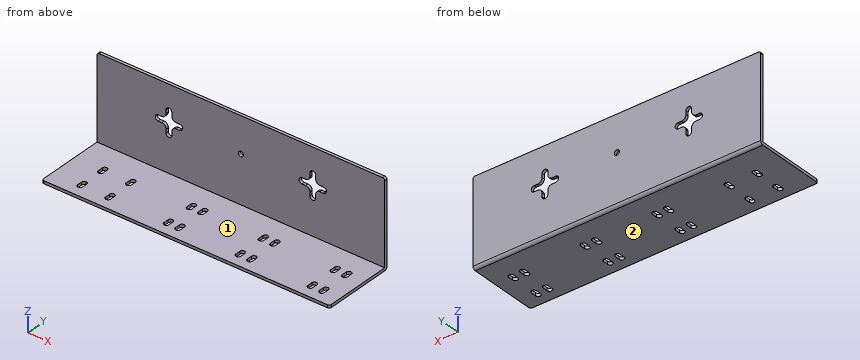
from build123d import *

# Parameters (mm, degrees)
F1_DEPTH = 100
F3_DEPTH = 60.001
F4_R     = 1.5
F5_R     = 2
F6_R     = 1.75
F6_W     = 2
F6_H     = 2
F7_DEPTH = 2
F8_R     = 3


with BuildPart() as f1:
    # F0 (on Right) → F1 (new body, symmetric)
    with BuildSketch(Plane.YZ):
        Polygon((0, 2), (0, 0), (50, 0), (50, 60), (48, 60), (48, 2), align=None)
    extrude(amount=F1_DEPTH, both=True)

    # F2 (on face) → F3 (cut, through all)
    with BuildSketch(Plane(origin=(0, 0, 0), x_dir=(1, 0, 0), z_dir=(0, 0, -1))):
        with BuildLine():
            Line((-18.25, -11.75), (-18.25, -10))
            Line((-18.25, -10), (-18.25, -8.25))
            ThreePointArc((-18.25, -8.25), (-20, -6.5), (-21.75, -8.25))
            Line((-21.75, -8.25), (-21.75, -11.75))
            ThreePointArc((-21.75, -11.75), (-20, -13.5), (-18.25, -11.75))
        make_face()
        with BuildLine():
            Line((-13.75, -8.25), (-13.75, -10))
            Line((-13.75, -10), (-13.75, -11.75))
            ThreePointArc((-13.75, -11.75), (-12, -13.5), (-10.25, -11.75))
            Line((-10.25, -11.75), (-10.25, -8.25))
            ThreePointArc((-10.25, -8.25), (-12, -6.5), (-13.75, -8.25))
        make_face()
        with BuildLine():
            ThreePointArc((-21.75, -31.75), (-20, -33.5), (-18.25, -31.75))
            Line((-18.25, -31.75), (-18.25, -28.25))
            ThreePointArc((-18.25, -28.25), (-20, -26.5), (-21.75, -28.25))
            Line((-21.75, -28.25), (-21.75, -31.75))
        make_face()
        with BuildLine():
            Line((-10.25, -31.75), (-10.25, -28.25))
            ThreePointArc((-10.25, -28.25), (-12, -26.5), (-13.75, -28.25))
            Line((-13.75, -28.25), (-13.75, -31.75))
            ThreePointArc((-13.75, -31.75), (-12, -33.5), (-10.25, -31.75))
        make_face()
        with BuildLine():
            Line((31.75, -10), (31.75, -8.25))
            ThreePointArc((31.75, -8.25), (30, -6.5), (28.25, -8.25))
            Line((28.25, -8.25), (28.25, -11.75))
            ThreePointArc((28.25, -11.75), (30, -13.5), (31.75, -11.75))
            Line((31.75, -11.75), (31.75, -10))
        make_face()
        with BuildLine():
            Line((39.75, -11.75), (39.75, -8.25))
            ThreePointArc((39.75, -8.25), (38, -6.5), (36.25, -8.25))
            Line((36.25, -8.25), (36.25, -10))
            Line((36.25, -10), (36.25, -11.75))
            ThreePointArc((36.25, -11.75), (38, -13.5), (39.75, -11.75))
        make_face()
        with BuildLine():
            Line((39.75, -31.75), (39.75, -28.25))
            ThreePointArc((39.75, -28.25), (38, -26.5), (36.25, -28.25))
            Line((36.25, -28.25), (36.25, -31.75))
            ThreePointArc((36.25, -31.75), (38, -33.5), (39.75, -31.75))
        make_face()
        with BuildLine():
            ThreePointArc((28.25, -31.75), (30, -33.5), (31.75, -31.75))
            Line((31.75, -31.75), (31.75, -28.25))
            ThreePointArc((31.75, -28.25), (30, -26.5), (28.25, -28.25))
            Line((28.25, -28.25), (28.25, -31.75))
        make_face()
        with BuildLine():
            Line((81.75, -10), (81.75, -8.25))
            ThreePointArc((81.75, -8.25), (80, -6.5), (78.25, -8.25))
            Line((78.25, -8.25), (78.25, -11.75))
            ThreePointArc((78.25, -11.75), (80, -13.5), (81.75, -11.75))
            Line((81.75, -11.75), (81.75, -10))
        make_face()
        with BuildLine():
            Line((89.75, -11.75), (89.75, -8.25))
            ThreePointArc((89.75, -8.25), (88, -6.5), (86.25, -8.25))
            Line((86.25, -8.25), (86.25, -10))
            Line((86.25, -10), (86.25, -11.75))
            ThreePointArc((86.25, -11.75), (88, -13.5), (89.75, -11.75))
        make_face()
        with BuildLine():
            ThreePointArc((78.25, -31.75), (80, -33.5), (81.75, -31.75))
            Line((81.75, -31.75), (81.75, -28.25))
            ThreePointArc((81.75, -28.25), (80, -26.5), (78.25, -28.25))
            Line((78.25, -28.25), (78.25, -31.75))
        make_face()
        with BuildLine():
            Line((89.75, -31.75), (89.75, -28.25))
            ThreePointArc((89.75, -28.25), (88, -26.5), (86.25, -28.25))
            Line((86.25, -28.25), (86.25, -31.75))
            ThreePointArc((86.25, -31.75), (88, -33.5), (89.75, -31.75))
        make_face()
        with BuildLine():
            ThreePointArc((-81.75, -11.75), (-81.2374368671, -12.9874368671), (-80, -13.5))
            ThreePointArc((-80, -13.5), (-78.7625631329, -12.9874368671), (-78.25, -11.75))
            Line((-78.25, -11.75), (-78.25, -8.25))
            ThreePointArc((-78.25, -8.25), (-80, -6.5), (-81.75, -8.25))
            Line((-81.75, -8.25), (-81.75, -11.75))
        make_face()
        with BuildLine():
            Line((-78.25, -29.75), (-78.25, -28))
            Line((-78.25, -28), (-78.25, -26.25))
            ThreePointArc((-78.25, -26.25), (-78.7625631329, -25.0125631329), (-80, -24.5))
            ThreePointArc((-80, -24.5), (-81.2374368671, -25.0125631329), (-81.75, -26.25))
            Line((-81.75, -26.25), (-81.75, -29.75))
            ThreePointArc((-81.75, -29.75), (-80, -31.5), (-78.25, -29.75))
        make_face()
        with BuildLine():
            Line((-62.35, -26.25), (-62.35, -28))
            Line((-62.35, -28), (-62.35, -29.75))
            ThreePointArc((-62.35, -29.75), (-60.6, -31.5), (-58.85, -29.75))
            Line((-58.85, -29.75), (-58.85, -26.25))
            ThreePointArc((-58.85, -26.25), (-60.6, -24.5), (-62.35, -26.25))
        make_face()
        with BuildLine():
            Line((-62.35, -10), (-62.35, -11.75))
            ThreePointArc((-62.35, -11.75), (-60.6, -13.5), (-58.85, -11.75))
            Line((-58.85, -11.75), (-58.85, -8.25))
            ThreePointArc((-58.85, -8.25), (-60.6, -6.5), (-62.35, -8.25))
            Line((-62.35, -8.25), (-62.35, -10))
        make_face()
    extrude(amount=-F3_DEPTH, mode=Mode.SUBTRACT)

    # F4
    f4_edges = [f1.edges().sort_by_distance(p)[0] for p in [
        (100, 0, 1),
        (100, 49, 60),
        (-100, 0, 1),
        (-100, 49, 60),
    ]]
    fillet(f4_edges, radius=F4_R)

    # F5
    f5_edges = [f1.edges().sort_by_distance(p)[0] for p in [
        (0, 50, 0),
    ]]
    fillet(f5_edges, radius=F5_R)

    # F6 (on face) → F7 (cut)
    with BuildSketch(Plane(origin=(0, 50, 0), x_dir=(-1, 0, 0), z_dir=(0, 1, 0))):
        with Locations((0, 35)):
            Circle(F6_R)
        with Locations((-49, 34)):
            Rectangle(F6_W, F6_H)
        with BuildLine():
            Line((-48, 37), (-48, 35))
            Line((-48, 35), (-48, 33))
            Line((-48, 33), (-42.5, 33))
            ThreePointArc((-42.5, 33), (-40.5, 35), (-42.5, 37))
            Line((-42.5, 37), (-48, 37))
        make_face()
        with Locations((-49, 36)):
            Rectangle(F6_W, F6_H)
        with Locations((-51, 34)):
            Rectangle(F6_W, F6_H)
        with Locations((-51, 36)):
            Rectangle(F6_W, F6_H)
        with BuildLine():
            Line((-48, 27.5), (-48, 33))
            Line((-48, 33), (-50, 33))
            Line((-50, 33), (-52, 33))
            Line((-52, 33), (-52, 27.5))
            ThreePointArc((-52, 27.5), (-50, 25.5), (-48, 27.5))
        make_face()
        with BuildLine():
            Line((-50, 37), (-48, 37))
            Line((-48, 37), (-48, 42.5))
            ThreePointArc((-48, 42.5), (-50, 44.5), (-52, 42.5))
            Line((-52, 42.5), (-52, 37))
            Line((-52, 37), (-50, 37))
        make_face()
        with BuildLine():
            Line((-52, 33), (-52, 35))
            Line((-52, 35), (-52, 37))
            Line((-52, 37), (-57.5, 37))
            ThreePointArc((-57.5, 37), (-59.5, 35), (-57.5, 33))
            Line((-57.5, 33), (-52, 33))
        make_face()
        with BuildLine():
            ThreePointArc((48, 27.5), (50, 25.5), (52, 27.5))
            Line((52, 27.5), (52, 33))
            Line((52, 33), (50, 33))
            Line((50, 33), (48, 33))
            Line((48, 33), (48, 27.5))
        make_face()
        with Locations((51, 34)):
            Rectangle(F6_W, F6_H)
        with BuildLine():
            Line((52, 35), (52, 33))
            Line((52, 33), (57.5, 33))
            ThreePointArc((57.5, 33), (59.5, 35), (57.5, 37))
            Line((57.5, 37), (52, 37))
            Line((52, 37), (52, 35))
        make_face()
        with Locations((51, 36)):
            Rectangle(F6_W, F6_H)
        with Locations((49, 34)):
            Rectangle(F6_W, F6_H)
        with BuildLine():
            Line((42.5, 33), (48, 33))
            Line((48, 33), (48, 35))
            Line((48, 35), (48, 37))
            Line((48, 37), (42.5, 37))
            ThreePointArc((42.5, 37), (40.5, 35), (42.5, 33))
        make_face()
        with BuildLine():
            Line((50, 37), (52, 37))
            Line((52, 37), (52, 42.5))
            ThreePointArc((52, 42.5), (50, 44.5), (48, 42.5))
            Line((48, 42.5), (48, 37))
            Line((48, 37), (50, 37))
        make_face()
        with Locations((49, 36)):
            Rectangle(F6_W, F6_H)
        with BuildLine():
            ThreePointArc((148, 27.5), (150, 25.5), (152, 27.5))
            Line((152, 27.5), (152, 33))
            Line((152, 33), (150, 33))
            Line((150, 33), (148, 33))
            Line((148, 33), (148, 27.5))
        make_face()
        with Locations((151, 34)):
            Rectangle(F6_W, F6_H)
        with BuildLine():
            Line((152, 35), (152, 33))
            Line((152, 33), (157.5, 33))
            ThreePointArc((157.5, 33), (159.5, 35), (157.5, 37))
            Line((157.5, 37), (152, 37))
            Line((152, 37), (152, 35))
        make_face()
        with Locations((151, 36)):
            Rectangle(F6_W, F6_H)
        with Locations((149, 34)):
            Rectangle(F6_W, F6_H)
        with BuildLine():
            Line((142.5, 33), (148, 33))
            Line((148, 33), (148, 35))
            Line((148, 35), (148, 37))
            Line((148, 37), (142.5, 37))
            ThreePointArc((142.5, 37), (140.5, 35), (142.5, 33))
        make_face()
        with BuildLine():
            Line((150, 37), (152, 37))
            Line((152, 37), (152, 42.5))
            ThreePointArc((152, 42.5), (150, 44.5), (148, 42.5))
            Line((148, 42.5), (148, 37))
            Line((148, 37), (150, 37))
        make_face()
        with Locations((149, 36)):
            Rectangle(F6_W, F6_H)
    extrude(amount=-F7_DEPTH, mode=Mode.SUBTRACT)

    # F8
    f8_edges = [f1.edges().sort_by_distance(p)[0] for p in [
        (52, 49, 33),
        (48, 49, 33),
        (48, 49, 37),
        (52, 49, 37),
        (-52, 49, 33),
        (-52, 49, 37),
        (-48, 49, 37),
        (-48, 49, 33),
    ]]
    fillet(f8_edges, radius=F8_R)


solid = f1.part
Work out the finished part from the listing and answer in its coordinate system (mm). Face numbers are marked on the shaded views. A direction names the side the tool comes from. Coordinates: 2 decimals unless noted, no trailing zeros. Write each loop counter-clockwise with the first axis right and the second up, starting at its lowest first coordinate (ties: lowest second). Pieces come first, ordered by that corner, then holes.
1. The part is cut by section B-B, the plane x = -20. Write down the section's boundary in (y, z), and give its area (3 significant figures).
Results list:
outline: (0, 0) - (6.5, 0) - (6.5, 2) - (0, 2) - close; (13.5, 0) - (26.5, 0) - (26.5, 2) - (13.5, 2) - close; (33.5, 0) - (48, 0) arc R2 ccw to (50, 2) - (50, 60) - (48, 60) - (48, 2) - (33.5, 2) - close
area: 187 mm2
2. The part is cut by section A-A, the plane z = 35. Write down the section's boundary in (x, y), and give its area (3 significant figures).
Results list:
outline: (-100, 48) - (-59.5, 48) - (-59.5, 50) - (-100, 50) - close; (-40.5, 48) - (-1.75, 48) - (-1.75, 50) - (-40.5, 50) - close; (1.75, 48) - (40.5, 48) - (40.5, 50) - (1.75, 50) - close; (59.5, 48) - (100, 48) - (100, 50) - (59.5, 50) - close
area: 317 mm2
3. Consider line 1 along Z through (x, y) = (0, 48.4); line 2 along Y through (x, z) = (-33.5, 57); line 3 along Z through (x, y) = (0, 49.35). Determine where each line is inside the solid, lowest interval first.
Results list:
line 1: z = 0.04 to 33.25, 36.75 to 60
line 2: y = 48 to 50
line 3: z = 0.52 to 33.25, 36.75 to 60
4. The part is cut by section C-C, the plane x = 0. Write down the section's boundary in (y, z), and give its area (3 significant figures).
Results list:
outline: (0, 0) - (48, 0) arc R2 ccw to (50, 2) - (50, 33.25) - (48, 33.25) - (48, 2) - (0, 2) - close; (48, 36.75) - (50, 36.75) - (50, 60) - (48, 60) - close
area: 208 mm2
5. For the marked faces 1 and 2, determine the directions among +Z, -Z, +X, -X, +Y, -Y from which every point of the face is accessible in a straight line to the end or side of a thin tool.
Results list:
face 1: +Z, +X, -X, -Y
face 2: -Z, +X, -X, +Y, -Y
6. Flat-ended cylindrical pins translate along their axes: pin 1 (1.6 mm diameter, centred on x = 43.5, y = 49, fed in from -Z); pin 2 (1.5 mm diameter, centred on x = -0.5, z = 36, fed in from -Y); pin 3 (2 mm diameter, centred on x = -57, y = 49.5, fed in from -Z). Find the tip coordinate at first contact, or state that the pin passes through.
Results list:
pin 1: stops at z = 0.01
pin 2: stops at y = 48
pin 3: stops at z = 0.06
7. The part is cut by section D-D, the plane x = 63.5. Write down the section's boundary in (y, z).
Results list:
outline: (0, 0) - (48, 0) arc R2 ccw to (50, 2) - (50, 60) - (48, 60) - (48, 2) - (0, 2) - close
